from build123d import *
from build123d.topology import SkipClean

# Parameters (mm, degrees)
BOSS_EXTRUDE1_DEPTH                             = 34.925
BOSS_EXTRUDE2_DEPTH                             = 38.1
CUT_EXTRUDE1_DEPTH                              = 28.575
FILLET1_START                                   = -6.35
FILLET1_DEPTH                                   = 6.35
BOSS_EXTRUDE3_START                             = -165.1
BOSS_EXTRUDE3_DEPTH                             = 57.15
SKETCH4_R                                       = 3.96875
CUT_EXTRUDE3_DEPTH                              = 232.143489097
CSK_FOR_12_FLAT_HEAD_MACHINE_SCREW1_D           = 5.7912
CSK_FOR_12_FLAT_HEAD_MACHINE_SCREW1_CSINK_D     = 11.1252
CSK_FOR_12_FLAT_HEAD_MACHINE_SCREW1_CSINK_ANGLE = 82


with BuildPart() as part:
    # Sketch2 → Boss-Extrude1 (new body)
    with BuildSketch(Plane(origin=(0, 0, 0), x_dir=(0, 0, -1), z_dir=(1, 0, 0))):
        with BuildLine():
            Line((28.575, -6.35), (0.398437524, -6.35))
            ThreePointArc((0.398437524, -6.35), (23.224782374, -42.664357172), (65.709887751, -48.562693987))
            Line((65.709887751, -48.562693987), (203.2, -6.35))
            Line((203.2, -6.35), (28.575, -6.35))
        make_face()
        Polygon((222.25, 0), (28.575, 0), (28.575, -6.35), (203.2, -6.35), (222.25, -6.35), align=None)
        with BuildLine():
            Line((28.575, 0), (0, 0))
            ThreePointArc((0, 0), (0.099707231, -3.181243957), (0.398437524, -6.35))
            Line((0.398437524, -6.35), (28.575, -6.35))
            Line((28.575, -6.35), (28.575, 0))
        make_face()
    boss_extrude1 = extrude(amount=BOSS_EXTRUDE1_DEPTH)

    # Sketch2<3> → Boss-Extrude2 (add)
    with BuildSketch(Plane(origin=(0, 0, 0), x_dir=(0, 0, -1), z_dir=(1, 0, 0))):
        Polygon((222.25, 0), (28.575, 0), (28.575, -6.35), (203.2, -6.35), (222.25, -6.35), align=None)
    boss_extrude2 = extrude(amount=BOSS_EXTRUDE2_DEPTH)

    # Sketch2<4> → Cut-Extrude1 (cut)
    with BuildSketch(Plane(origin=(0, 0, 0), x_dir=(0, 0, -1), z_dir=(1, 0, 0))):
        with BuildLine():
            Line((28.575, -6.35), (0.398437524, -6.35))
            ThreePointArc((0.398437524, -6.35), (23.224782374, -42.664357172), (65.709887751, -48.562693987))
            Line((65.709887751, -48.562693987), (203.2, -6.35))
            Line((203.2, -6.35), (28.575, -6.35))
        make_face()
    cut_extrude1 = extrude(amount=CUT_EXTRUDE1_DEPTH, mode=Mode.SUBTRACT)

    # Fillet1: read off the stored shape, not the designer's step
    # Fillet1 outline → Fillet1 (add)
    with BuildSketch(Plane(origin=(0, 0, 0), x_dir=(1, 0, 0), z_dir=(0, 1, 0)).offset(FILLET1_START)):
        with BuildLine():
            Line((34.925, 28.575), (34.925, 16.278277876))
            add(Edge.make_bspline(
                [(34.925, 16.278277876), (34.925, 22.836529675), (38.1, 28.575)],
                knots=[0, 0, 0, 1, 1, 1], degree=2, weights=[1, 1.936491673, 1]))
            Line((38.1, 28.575), (34.925, 28.575))
        make_face()
    fillet1 = extrude(amount=FILLET1_DEPTH)

    # Sketch3 → Boss-Extrude3 (add)
    with BuildSketch(Plane(origin=(0, 0, -222.25), x_dir=(-1, 0, 0), z_dir=(0, 0, -1)).offset(BOSS_EXTRUDE3_START)):
        with BuildLine():
            Line((0, 0), (0, 3.175))
            ThreePointArc((0, 3.175), (-12.7, 15.875), (0, 28.575))
            Line((0, 28.575), (0, 38.1))
            ThreePointArc((0, 38.1), (-13.852256532, 33.255034924), (-21.665035078, 20.832507443))
            ThreePointArc((-21.665035078, 20.832507443), (-24.250245873, 15.107068484), (-28.853915615, 10.832704084))
            ThreePointArc((-28.853915615, 10.832704084), (-33.303746055, 6.208976231), (-34.925, 0))
            Line((-34.925, 0), (0, 0))
        make_face()
    boss_extrude3 = extrude(amount=-BOSS_EXTRUDE3_DEPTH)

    # Mirror1: Boss-Extrude1, Boss-Extrude2, Cut-Extrude1, Fillet1, Boss-Extrude3 across plane
    with SkipClean():  # the faces are left unmerged after this step: merging them gives an invalid solid
        add(boss_extrude1.mirror(Plane(origin=(0, 28.575, 0), x_dir=(0, 0, 1), z_dir=(-1, 0, 0))))
        add(boss_extrude2.mirror(Plane(origin=(0, 28.575, 0), x_dir=(0, 0, 1), z_dir=(-1, 0, 0))))
        add(cut_extrude1.mirror(Plane(origin=(0, 28.575, 0), x_dir=(0, 0, 1), z_dir=(-1, 0, 0))), mode=Mode.SUBTRACT)
        add(fillet1.mirror(Plane(origin=(0, 28.575, 0), x_dir=(0, 0, 1), z_dir=(-1, 0, 0))))
        add(boss_extrude3.mirror(Plane(origin=(0, 28.575, 0), x_dir=(0, 0, 1), z_dir=(-1, 0, 0))))

    # Sketch4 → Cut-Extrude3 (cut, through all)
    with SkipClean():  # the faces are left unmerged after this step: merging them gives an invalid solid
        with BuildSketch(Plane(origin=(0, 0, 0), x_dir=(1, 0, 0), z_dir=(0, 1, 0))):
            with Locations(Location((0, 203.2, 0), (0, 0, 270))):
                Circle(SKETCH4_R)
            with Locations(Location((0, 139.7, 0), (0, 0, 270))):
                Circle(SKETCH4_R)
            with Locations(Location((0, 76.2, 0), (0, 0, 270))):
                Circle(SKETCH4_R)
        extrude(amount=-CUT_EXTRUDE3_DEPTH, mode=Mode.SUBTRACT)

    # CSK for #12 Flat Head Machine Screw1 (through all)
    with Locations(Plane(origin=(0, 0, 0), x_dir=(1, 0, 0), z_dir=(0, 1, 0))):
        with Locations((0, 76.2), (0, 139.7), (0, 203.2)):
            CounterSinkHole(CSK_FOR_12_FLAT_HEAD_MACHINE_SCREW1_D / 2, CSK_FOR_12_FLAT_HEAD_MACHINE_SCREW1_CSINK_D / 2, counter_sink_angle=CSK_FOR_12_FLAT_HEAD_MACHINE_SCREW1_CSINK_ANGLE)


solid = part.part
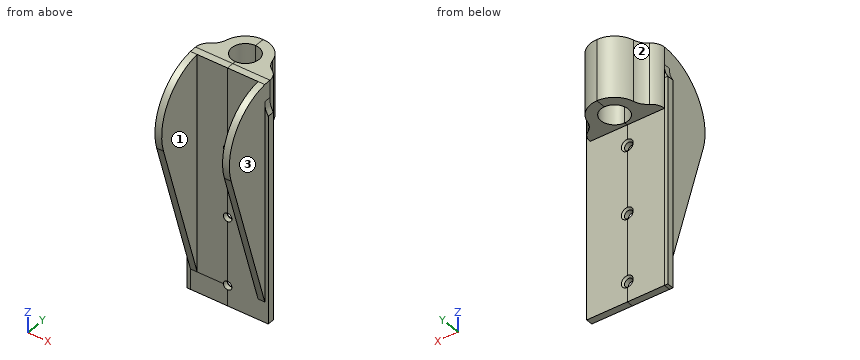
Verification items for the finished model (mm, model axes). Face numbers are marked on the shaded views. Round coordinates to 2 decimals unless told otherwise and drop trailing zeros. Loops run counter-clockwise (first coordinate to the right, second up) from the corner with the lowest first, then second, coordinate; pieces in that order, holes last. Notation, with made-up numbers: (79, 68) - (108, 68) arc R19 ccw to (108, 97) - close; hole circle Ø6 at (44.25, 2). An arc over 180 degrees is marked (long way). Use one line per item in the form item = value.
1. Section check A-A on z = -76.2. Record the cut outline in (x, y) (3 decimals), and give its area (3 significant figures).
A:
outline = (-38.1, -6.35) - (-34.925, -6.35) - (-34.925, -45.342) - (-28.575, -45.342) - (-28.575, -6.35) - (-3.969, -6.35) - (-3.969, -1.834) - (-5.563, 0) - (-38.1, 0) - close; (3.969, -6.35) - (28.575, -6.35) - (28.575, -45.342) - (34.925, -45.342) - (34.925, -6.35) - (38.1, -6.35) - (38.1, 0) - (5.563, 0) - (3.969, -1.834) - close
area = 926 mm²
2. Section check C-C on x = 17. Record the cut outline in (y, z).
A:
outline = (-6.35, -222.25) - (0, -222.25) - (0, -57.15) - (30.19, -57.15) - (30.19, 0) - (0, 0) arc R50.8 ccw to (-6.35, -0.4) - close
3. Gauge pin test, flat ends, axial feed: pin 1 Ø12 at (y, z) = (19.5, -28) entering from -X; pin 2 Ø3.5 at (x, z) = (-36, -143.5) entering from -Y; pin 3 Ø4 at (x, z) = (21.5, -102.5) entering from -Y. Record the tip position at first contact, or that the pin passes through.
A:
pin_1 = -25.57
pin_2 = -25.1
pin_3 = -6.35
4. Section check D-D on x = -8. Record the cut outline in (y, z).
A:
outline = (-6.35, -222.25) - (0, -222.25) - (0, -57.15) - (6.01, -57.15) - (6.01, 0) - (0, 0) arc R50.8 ccw to (-6.35, -0.4) - close; (25.74, -57.15) - (36.61, -57.15) - (36.61, 0) - (25.74, 0) - close
5. Scan lines: probe 1 along X at (y, z) = (-32.5, -54) (3 decimals); probe 2 along X at (y, z) = (-4.55, -203.2); probe 3 along Z at (x, y) = (0, -3). Record each from-to range of solid material in increasing order.
A:
probe_1 = -34.925 to -28.575, 28.575 to 34.925
probe_2 = -38.1 to -3.97, 3.97 to 38.1
probe_3 = -222.25 to -207.17, -199.23 to -143.67, -135.73 to -80.17, -72.23 to -0.09
6. Section check B-B on y = -21. Record the cut outline in (x, z) (3 decimals).
A:
outline = (-34.925, -155.484) - (-28.575, -155.484) - (-28.575, -4.544) - (-34.925, -4.544) - close; (28.575, -155.484) - (34.925, -155.484) - (34.925, -4.544) - (28.575, -4.544) - close
7. Draft check along X on the marked faces 1, 2 and 3. Enter one of: pulls with the +X half, pulls with the -X half, needs draft (parallel to the pull), parting line crosses it, or undercut.
A:
face_1 = undercut
face_2 = pulls with the -X half
face_3 = pulls with the +X half
